from build123d import *

# Parameters (mm, degrees)
SKETCH1_R           = 1.1938
BOSS_EXTRUDE1_DEPTH = 7.7724


with BuildPart() as part:
    # Sketch1 → Boss-Extrude1 (new body)
    with BuildSketch(Plane.XY):
        with BuildLine():
            Line((-5.065262452, 5.08), (-18.456556559, 5.08))
            ThreePointArc((-18.456556559, 5.08), (-19.426909517, 4.731155792), (-19.953034117, 3.844324324))
            ThreePointArc((-19.953034117, 3.844324324), (-18.44069754, -8.534815418), (-9.9822, -17.699098371))
            Line((-9.9822, -17.699098371), (-9.9822, -16.784328658))
            Line((-9.9822, -16.784328658), (2.593084415, -20.153865962))
            ThreePointArc((2.593084415, -20.153865962), (13.682234942, -15.023276839), (19.824330155, -4.46075486))
            Line((19.824330155, -4.46075486), (17.325781624, -1.483100672))
            ThreePointArc((17.325781624, -1.483100672), (17.037851626, -1.347023051), (16.747173773, -1.477127579))
            ThreePointArc((16.747173773, -1.477127579), (11.324901076, -3.317959511), (7.028137334, 0.467212181))
            Line((7.028137334, 0.467212181), (6.053096787, 3.371693793))
            ThreePointArc((6.053096787, 3.371693793), (1.669604011, 7.303273092), (-3.95481445, 5.560217822))
            ThreePointArc((-3.95481445, 5.560217822), (-4.460344292, 5.205196933), (-5.065262452, 5.08))
        make_face()
        with Locations((15.748, -5.08)):
            Circle(SKETCH1_R, mode=Mode.SUBTRACT)
        with BuildLine():
            Line((-3.876453526, 1.038692592), (-3.482013301, 2.510763551))
            ThreePointArc((-3.482013301, 2.510763551), (-2.298514325, 4.447599489), (-0.253578298, 5.432607064))
            Line((-0.253578298, 5.432607064), (-0.201054745, 5.628627633))
            ThreePointArc((-0.201054745, 5.628627633), (-0.082709585, 5.782858048), (0.110030452, 5.808232755))
            Line((0.110030452, 5.808232755), (2.808827211, 5.085092343))
            ThreePointArc((2.808827211, 5.085092343), (2.963057626, 4.966747183), (2.988432333, 4.774007146))
            Line((2.988432333, 4.774007146), (2.93590878, 4.577986577))
            ThreePointArc((2.93590878, 4.577986577), (4.214371541, 2.702476981), (4.270893751, 0.433378367))
            Line((4.270893751, 0.433378367), (3.876453526, -1.038692592))
            ThreePointArc((3.876453526, -1.038692592), (-1.038692592, -3.876453526), (-3.876453526, 1.038692592))
        make_face(mode=Mode.SUBTRACT)
    extrude(amount=-BOSS_EXTRUDE1_DEPTH)


solid = part.part
The model under review builds one solid part; all positions refer to its coordinate system, in mm. A direction names the side the tool comes from. Round coordinates to 2 decimals unless told otherwise and drop trailing zeros. Write each loop counter-clockwise with the first axis right and the second up, starting at its lowest first coordinate (ties: lowest second). Pieces come first, ordered by that corner, then holes. Notation, with made-up numbers: (86.25, 45) -> (134.25, 45) arc R34 ccw to (134.25, 84) -> close; hole circle Ø4 at (56.25, 53). An arc over 180 degrees is marked (long way). Answer as a JSON object with one key per item and string values.
1. To check wall thickness, follow line 1 along X through (y, z) = (-2, -2.5); line 2 along Y through (x, z) = (0, -6); line 3 along X through (y, z) = (0.5, -3). State the ranges of each line that lie inside material, in increasing order.
Results found:
{"line 1": "x = -20.22 to -3.48, 3.48 to 8.67, 16.23 to 17.76", "line 2": "y = -19.46 to -4.01, 5.81 to 7.43", "line 3": "x = -20.31 to -3.98, 4.29 to 7.02"}
2. We need section D-D on x = -6.5. State the section outline as (y, z) points, and give its area (3 significant figures).
Results found:
{"outline": "(-17.72, -7.77) -> (5.08, -7.77) -> (5.08, 0) -> (-17.72, 0) -> close", "area": "177 mm^2"}
3. The part is to be moulded in two halves that separate along X. For faces 4 (the face through (18.6, -3, -3.8)), 5 (the face through (-1, -6, -7.772)), 6 (the face through (-2.32, 4.43, -3.83)), 7 (the face through (15.489, -6.245, -3.832)), say which applies: pulls with the +X half, pulls with the -X half, needs draft (parallel to the pull), parting line crosses it, or undercut.
Results found:
{"face 4": "pulls with the +X half", "face 5": "needs draft", "face 6": "undercut", "face 7": "undercut"}
4. Machinability: for faces 1 (the face through (13.6, -15.1, -3.8)), 2 (the face through (-12, 5.08, -4)), 3 (the face through (-3.682, 1.764, -3.832)), which of the approach directions +Z, -Z, +X, -X, +Y, -Y give a long, thin tool a straight path to every point of the face, cutting with its end or side? Answer none if there is none.
Results found:
{"face 1": "+Z, -Z, +X, -Y", "face 2": "+Z, -Z, -X, +Y", "face 3": "+Z, -Z"}
5. We need section C-C on y = 0. State the section outline as (x, z) points.
Results found:
{"outline": "(-20.32, -7.77) -> (-4.01, -7.77) -> (-4.01, 0) -> (-20.32, 0) -> close; (4.15, -7.77) -> (7.21, -7.77) -> (7.21, 0) -> (4.15, 0) -> close"}
6. We need section A-A on z = -4.5. State the section outline as (x, y) points (3 decimals), and give its area (3 significant figures).
Results found:
{"outline": "(-19.953, 3.844) arc R20.32 ccw to (-9.982, -17.699) -> (-9.982, -16.784) -> (2.593, -20.154) arc R20.32 ccw to (19.824, -4.461) -> (17.326, -1.483) arc R0.381 ccw to (16.747, -1.477) arc R5.715 cw to (7.028, 0.467) -> (6.053, 3.372) arc R5.969 ccw to (-3.955, 5.56) arc R1.524 cw to (-5.065, 5.08) -> (-18.457, 5.08) arc R1.524 ccw to start; hole (-3.876, 1.039) arc R4.013 ccw to (3.876, -1.039) -> (4.271, 0.433) arc R4.013 ccw to (2.936, 4.578) -> (2.988, 4.774) arc R0.254 ccw to (2.809, 5.085) -> (0.11, 5.808) arc R0.254 ccw to (-0.201, 5.629) -> (-0.254, 5.433) arc R4.013 ccw to (-3.482, 2.511) -> close; hole circle Ø2.388 at (15.748, -5.08)", "area": "681 mm^2"}
7. Clearance check with flat-ended pins moving along their axes: pin 1 (2 mm diameter, centred on x = -2.5, z = -4.5, fed in from -Y); pin 2 (1.9 mm diameter, centred on x = 15.748, y = -5.08, fed in from -Z); pin 3 (1.5 mm diameter, centred on y = -8, z = -6, fed in from +X); pin 4 (3 mm diameter, centred on x = -11, z = -6, fed in from +Y). State where each tip first meets the part, or that it passes through.
Results found:
{"pin 1": "stops at y = -19.06", "pin 2": "passes through", "pin 3": "stops at x = 18.98", "pin 4": "stops at y = 5.08"}
8. We need section B-B on y = -5.08. State the section outline as (x, z) points.
Results found:
{"outline": "(-19.67, -7.77) -> (14.55, -7.77) -> (14.55, 0) -> (-19.67, 0) -> close; (16.94, -7.77) -> (19.67, -7.77) -> (19.67, 0) -> (16.94, 0) -> close"}
